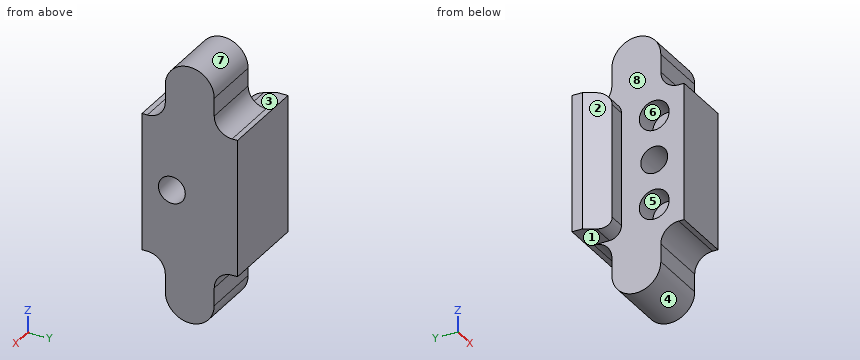
```python
from build123d import *

# Parameters (mm, degrees)
EXTRUDE_1_DEPTH          = 23
SKETCH_2_R               = 2.5
CUT_EXTRUDE_1_DEPTH      = 4
CUT_EXTRUDE_1_DEPTH_BACK = 30.774100013
HOLE_WIZARD_M41_D        = 4.5
CHAMFER_1_SIZE           = 1
CHAMFER_1_SIZE2          = 2
EXTRUDE_2_DEPTH          = 10.074573519
FILLET_1_R               = 3
FILLET_2_R               = 2


with BuildPart() as part:
    # Эскиз1 → Бобышка-Вытянуть1 (new body)
    with BuildSketch(Plane.XY):
        Polygon((0, 0), (-10.074573519, 0), (-10.074573519, 10.5), (-12.824573519, 10.5), (-16, 16), (0, 16), align=None)
    extrude(amount=EXTRUDE_1_DEPTH)

    # Эскиз2 → Вырез-Вытянуть1 (cut, two sides)
    with BuildSketch(Plane(origin=(-10.074573519, 0, 0), x_dir=(0, 0, -1), z_dir=(1, 0, 0))) as cut_extrude_1_sk:
        with Locations((-19, 5)):
            Circle(SKETCH_2_R)
        with Locations(Location((-4, 5, 0), (0, 0, 90))):
            Circle(SKETCH_2_R)
    extrude(amount=CUT_EXTRUDE_1_DEPTH, mode=Mode.SUBTRACT)
    extrude(cut_extrude_1_sk.sketch, amount=-CUT_EXTRUDE_1_DEPTH_BACK, mode=Mode.SUBTRACT)

    # Отверстие с зазором M41 (through all)
    with Locations(Plane(origin=(0, 1.542761086, 4.525415006), x_dir=(0, 0, 1), z_dir=(1, 0, 0))):
        with Locations((6.974584994, -3.457238914)):
            Hole(HOLE_WIZARD_M41_D / 2)

    # Фаска1
    chamfer_1_edges = [part.edges().sort_by_distance(p)[0] for p in [
        (-16, 16, 11.5),
    ]]
    chamfer_1_side = [part.faces().sort_by_distance(p)[0] for p in [
        (-8, 16, 11.5),
    ]]
    chamfer(chamfer_1_edges, length=CHAMFER_1_SIZE, length2=CHAMFER_1_SIZE2, reference=chamfer_1_side[0])

    # Эскиз7 → Бобышка-Вытянуть2 (add)
    with BuildSketch(Plane.ZY):
        with BuildLine():
            Line((-6, 12.1), (0, 12.1))
            Line((0, 12.1), (0, 3.9))
            Line((0, 3.9), (-6, 3.9))
            ThreePointArc((-6, 3.9), (-10.1, 8), (-6, 12.1))
        make_face()
        with BuildLine():
            Line((23, 12.1), (23, 3.9))
            Line((23, 3.9), (29, 3.9))
            ThreePointArc((29, 3.9), (33.1, 8), (29, 12.1))
            Line((29, 12.1), (23, 12.1))
        make_face()
    extrude(amount=EXTRUDE_2_DEPTH)

    # Скругление1
    fillet_1_edges = [part.edges().sort_by_distance(p)[0] for p in [
        (-5.037286759, 3.9, 23),
        (-5.03728676, 12.1, 23),
        (-5.03728676, 12.1, 0),
        (-5.037286759, 3.9, 0),
    ]]
    fillet(fillet_1_edges, radius=FILLET_1_R)

    # Скругление2
    fillet_2_edges = [part.edges().sort_by_distance(p)[0] for p in [
        (-11.449573519, 10.5, 23),
        (-11.449573519, 10.5, 0),
    ]]
    fillet(fillet_2_edges, radius=FILLET_2_R)


solid = part.part
```
Could you check a few things on this model? Use its own coordinates, in mm. Face numbers are marked on the shaded views. A direction names the side the tool comes from. Coordinates: 2 decimals unless noted, no trailing zeros. Write each loop counter-clockwise with the first axis right and the second up, starting at its lowest first coordinate (ties: lowest second). Pieces come first, ordered by that corner, then holes. Notation, with made-up numbers: (59.25, 24) -> (101.25, 24) arc R32 ccw to (101.25, 60) -> close; hole circle Ø6 at (-37, 77.25). An arc over 180 degrees is marked (long way). Write item = value, one per line. Start each with the question number.
(1) I want a section at A-A (z = 11.5). Please give me the cut outline in (x, y).
(2) I need wall thicknesses on line 1 (Y direction, x = -7.65, z = 19); line 2 (Z direction, x = -14, y = 14.75); line 3 (X direction, y = 6, z = 8). Which ranges of each line are inside material? Lowest first, please. Write a range as [from, to].
(3) I want a section at D-D (x = -7). Please give me the cut outline in (y, z).
(4) Which directions (+Z, -Z, +X, -X, +Y, -Y) give clear straight access to the entire face, cutting with the end or side of a thin tool? Please do the marked faces 1, 2, 3, 4 and 5.
(5) I want a section at C-C (y = 5). Please give me the cut outline in (x, z).
(6) Will these pins go through, and if not, where does the flat tip stop? pin 1 (7 mm diameter, centred on y = 5, z = 11.5, fed in from -X); pin 2 (4.5 mm diameter, centred on y = 10, z = 17.5, fed in from -X); pin 3 (1.5 mm diameter, centred on x = -6.5, z = 27.5, fed in from +Y).
(7) I want a section at B-B (x = -2). Please give me the cut outline in (y, z).
(8) We'd pull the mould along Z, two halves only. Please class the marked faces 6, 7 and 8: released by +Z, released by -Z, zero draft, split by the parting line, or undercut.
Result set:
q1.outline = (-15, 14.27) -> (-12.82, 10.5) -> (-10.07, 10.5) -> (-10.07, 7.25) -> (0, 7.25) -> (0, 16) -> (-15, 16) -> close; (-10.07, 0) -> (0, 0) -> (0, 2.75) -> (-10.07, 2.75) -> close
q2.line_1 = [0, 2.5], [7.5, 16]
q2.line_2 = [0, 23]
q2.line_3 = [-10.07, 0]
q3.outline = (0, 0) -> (0.9, 0) arc R3 cw to (3.9, -3) -> (3.9, -6) arc R4.1 ccw to (12.1, -6) -> (12.1, -3) arc R3 cw to (15.1, 0) -> (16, 0) -> (16, 23) -> (15.1, 23) arc R3 cw to (12.1, 26) -> (12.1, 29) arc R4.1 ccw to (3.9, 29) -> (3.9, 26) arc R3 cw to (0.9, 23) -> (0, 23) -> close; hole circle Ø5 at (5, 4); hole circle Ø5 at (5, 19); hole circle Ø4.5 at (5, 11.5)
q4.face_1 = -Z, -X, +Y
q4.face_2 = +Z, -Z, -X, -Y
q4.face_3 = +Z, -X, +Y
q4.face_4 = -Z, +X, -X
q4.face_5 = -X
q5.outline = (-10.07, -8.79) -> (0, -8.79) -> (0, 9.25) -> (-10.07, 9.25) -> (-10.07, 6.5) -> (-6.07, 6.5) -> (-6.07, 1.5) -> (-10.07, 1.5) -> close; (-10.07, 13.75) -> (0, 13.75) -> (0, 31.79) -> (-10.07, 31.79) -> (-10.07, 21.5) -> (-6.07, 21.5) -> (-6.07, 16.5) -> (-10.07, 16.5) -> close
q6.pin_1 = -10.07
q6.pin_2 = -13.83
q6.pin_3 = 12.1
q7.outline = (0, 0) -> (0.9, 0) arc R3 cw to (3.9, -3) -> (3.9, -6) arc R4.1 ccw to (12.1, -6) -> (12.1, -3) arc R3 cw to (15.1, 0) -> (16, 0) -> (16, 23) -> (15.1, 23) arc R3 cw to (12.1, 26) -> (12.1, 29) arc R4.1 ccw to (3.9, 29) -> (3.9, 26) arc R3 cw to (0.9, 23) -> (0, 23) -> close; hole circle Ø4.5 at (5, 11.5)
q8.face_6 = undercut
q8.face_7 = released by +Z
q8.face_8 = zero draft
